Geometry: final body of the model. Coordinates: model frame, mm. Face numbers are marked on the shaded views. A direction names the side the tool comes from. Round coordinates to 2 decimals unless told otherwise and drop trailing zeros. Order: outer loops, then holes, each group sorted by start corner. A loop starts at its lowest first (then second) coordinate and runs counter-clockwise, first axis right, second up. Notation, with made-up numbers: M -0.5,-15.5 L 28.5,-15.5 A9 ccw 28.5,-8.5 Z; hole C 22.5,89.5 d7. An arc over 180 degrees is marked long. Put each result on its own line as item: value. Start each with the question number.
1) Material intervals for probe 1 along X at (y, z) = (0, 10); probe 2 along X at (y, z) = (0, -7); probe 3 along X at (y, z) = (-4, -12.5), sorted ascending. Write a range as [from, to].
2) Access query for the marked faces 1 and 2. Directions: +Z, -Z, +X, -X, +Y, -Y. A direction counts if a zero-diameter tool reaches every point of the face in a straight line with its end or side. Return the directions, or none.
3) Section C-C, the plane z = 10. Count the separate pieces of the cut face and the enclosed holes in it, then the cut area to 3 significant figures.
4) Section D-D, the plane x = 43. Return loops of the section in (y, z), then the cut area to 3 significant figures.
5) Section B-B, the plane x = -57. Return loops of the section in (y, z).
6) Section A-A, the plane y = 0. Return loops of the section in (x, z), then the cut area to 3 significant figures.
7) First-contact query: P1, Ø4, axis at x = 60.5, y = 12, coming from the -Z side; P2, Ø2, axis at x = -6, z = -5, coming from the -Y side; P3, Ø1.5, axis at x = 7, z = -11.5, coming from the -Y side; P4, Ø5.5, axis at x = -30, y = 0, coming from the -Z side. Flat tips, straight axial feed; report the tip coordinate or a pass-through.
from build123d import *

# Parameters (mm, degrees)
SKETCH_1_R               = 12.5
EXTRUDE_1_DEPTH          = 75
SKETCH_2_R               = 15
EXTRUDE_2_DEPTH          = 70
CHAMFER_1_SIZE           = 1
CUT_EXTRUDE_1_DEPTH      = 4
SKETCH_4_R               = 3
CUT_EXTRUDE_2_DEPTH      = 16
CUT_EXTRUDE_2_DEPTH_BACK = 16


with BuildPart() as part:
    # 草图1 → 凸台-拉伸1 (new body)
    with BuildSketch(Plane(origin=(0, 0, 0), x_dir=(0, 0, -1), z_dir=(1, 0, 0))):
        Circle(SKETCH_1_R)
    extrude(amount=EXTRUDE_1_DEPTH)

    # 草图2 → 凸台-拉伸2 (add)
    with BuildSketch(Plane.ZY):
        Circle(SKETCH_2_R)
    extrude(amount=EXTRUDE_2_DEPTH)

    # 倒角1
    chamfer_1_edges = [part.edges().sort_by_distance(p)[0] for p in [
        (75, 0, 12.5),
        (0, 0, -15),
        (-70, 0, -15),
    ]]
    chamfer(chamfer_1_edges, length=CHAMFER_1_SIZE)

    # 草图3 → 切除-拉伸1 (cut)
    with BuildSketch(Plane.XY.offset(12.5)):
        with BuildLine():
            Line((32.999999837, 4), (68.999998276, 4))
            ThreePointArc((68.999998276, 4), (73, 5.01e-07), (68.999999277, -4))
            Line((68.999999277, -4), (33.000000086, -4))
            ThreePointArc((33.000000086, -4), (29, -1.25e-07), (32.999999837, 4))
        make_face()
    extrude(amount=-CUT_EXTRUDE_1_DEPTH, mode=Mode.SUBTRACT)

    # 草图4 → 切除-拉伸2 (cut, two sides)
    with BuildSketch(Plane.XY) as cut_extrude_2_sk:
        with Locations((-30, 0)):
            Circle(SKETCH_4_R)
    extrude(amount=CUT_EXTRUDE_2_DEPTH, mode=Mode.SUBTRACT)
    extrude(cut_extrude_2_sk.sketch, amount=-CUT_EXTRUDE_2_DEPTH_BACK, mode=Mode.SUBTRACT)


solid = part.part
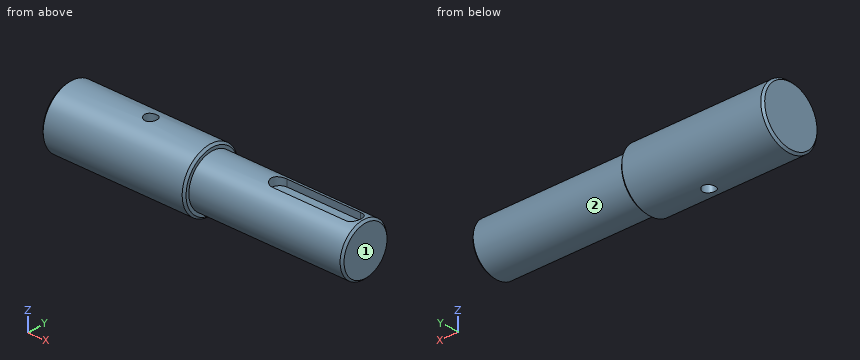
Result sheet:
1. probe 1: x = [-70, -33], [-27, 29], [73, 75]
1. probe 2: x = [-70, -33], [-27, 75]
1. probe 3: x = [-70, 0]
2. face 1: +Z, -Z, +X, +Y, -Y
2. face 2: +X
3. separate pieces: 1
3. enclosed holes: 2
3. area: 2,320 mm2
4. outline: M -4,8.5 L -4,11.84 A12.5 ccw long 4,11.84 L 4,8.5 Z
4. area: 461 mm2
5. outline: C 0,0 d30
6. outline: M -70,-14 L -69,-15 L -33,-15 L -33,15 L -69,15 L -70,14 Z; M -27,-15 L -1,-15 L 0,-14 L 0,-12.5 L 74,-12.5 L 75,-11.5 L 75,11.5 L 74,12.5 L 73,12.5 L 73,8.5 L 29,8.5 L 29,12.5 L 0,12.5 L 0,14 L -1,15 L -27,15 Z
6. area: 3,620 mm2
7. P1: stops at z = -7.5
7. P2: stops at y = -14.46
7. P3: stops at y = -6.38
7. P4: passes through
